Could you check a few things on this drawing? It's one solid part, dimensions in mm from its lowest x, y, z. A direction names the side the tool comes from. Give positions to 0.01 mm unless a question says otherwise; leave off trailing zeros. Order: outer loops, then holes, each group sorted by start corner. A loop starts at its lowest first (then second) coordinate and runs counter-clockwise, first axis right, second up. Notation, with made-up numbers: (14.5, -39.5) - (35.5, -39.5) arc R6 ccw to (35.5, -35.5) - close; hole circle Ø4 at (-29, -38.75). An arc over 180 degrees is marked (long way). One line per question, with ' | ' between items. Start each with the question number.
1. I need wall thicknesses on probe 1 along X at (y, z) = (2.85, 5.1); probe 2 along Z at (x, y) = (5.1, 0.2). Which ranges of each line are inside material? Lowest first, please. Write a range as from..to.
2. Imagine slicing it at B-B (z = 5.1). Please give me the cut outline in (x, y).
3. Imagine slicing it at A-A (x = 5.1). Please give me the cut outline in (y, z), and give its area (3 significant figures).
4. If we mould it in two halves opening along Z, with no side actions, what happens to the marked faces 1, 2 and 3? For each: released by +Z, released by -Z, zero draft, split by the parting line, or undercut.
5. Which directions (+Z, -Z, +X, -X, +Y, -Y) give clear straight access to the entire face, cutting with the end or side of a thin tool? Please do the marked faces 4 and 5.
6. Imagine slicing it at D-D (z = 8.5). Please give me the cut outline in (x, y), and give its area (3 significant figures).
7. Imagine slicing it at C-C (y = 0.6). Please give me the cut outline in (x, z).
8. For P1, Ø3, axis at x = 4.5, z = 5.5, coming from the -Y side; P2, Ø1.5, axis at x = 2, y = 1.5, coming from the -Z side; P3, Ø1, axis at x = 3, z = 7.5, coming from the -Y side; P4, Ø1, axis at y = 2.5, z = 7.5, coming from the +X side, each with a flat end and sliding along its axis, tell me the tip position at first contact or that it passes through.
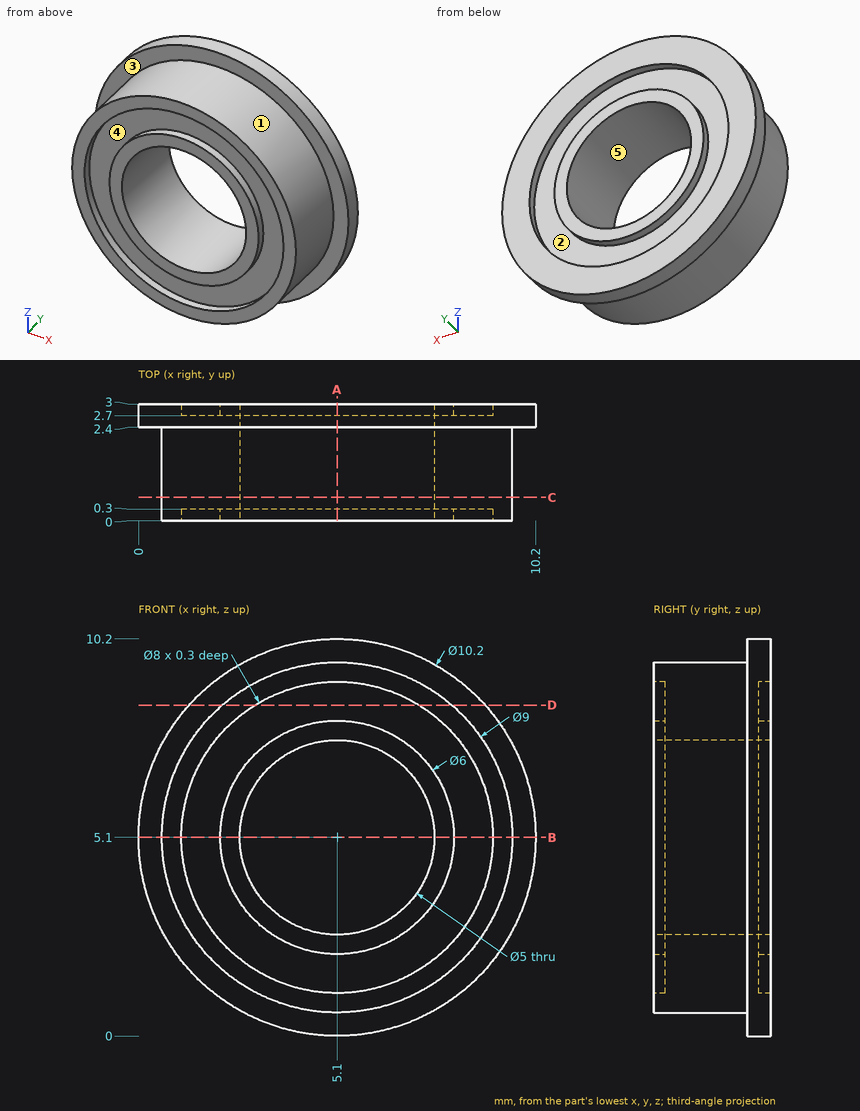
Results found:
1) probe 1: x = 0..1.1, 2.1..2.6, 7.6..8.1, 9.1..10.2 | probe 2: z = 0.6..1.1, 2.1..2.6, 7.6..8.1, 9.1..9.6
2) outline: (0, 2.4) - (0.6, 2.4) - (0.6, 0) - (1.1, 0) - (1.1, 0.3) - (2.1, 0.3) - (2.1, 0) - (2.6, 0) - (2.6, 3) - (2.1, 3) - (2.1, 2.7) - (1.1, 2.7) - (1.1, 3) - (0, 3) - close; (7.6, 0) - (8.1, 0) - (8.1, 0.3) - (9.1, 0.3) - (9.1, 0) - (9.6, 0) - (9.6, 2.4) - (10.2, 2.4) - (10.2, 3) - (9.1, 3) - (9.1, 2.7) - (8.1, 2.7) - (8.1, 3) - (7.6, 3) - close
3) outline: (0, 0.6) - (2.4, 0.6) - (2.4, 0) - (3, 0) - (3, 1.1) - (2.7, 1.1) - (2.7, 2.1) - (3, 2.1) - (3, 2.6) - (0, 2.6) - (0, 2.1) - (0.3, 2.1) - (0.3, 1.1) - (0, 1.1) - close; (0, 7.6) - (3, 7.6) - (3, 8.1) - (2.7, 8.1) - (2.7, 9.1) - (3, 9.1) - (3, 10.2) - (2.4, 10.2) - (2.4, 9.6) - (0, 9.6) - (0, 9.1) - (0.3, 9.1) - (0.3, 8.1) - (0, 8.1) - close | area: 11.5 mm2
4) face 1: split by the parting line | face 2: undercut | face 3: zero draft
5) face 4: -Y | face 5: +Y, -Y
6) outline: (1.3, 2.4) - (2.15, 2.4) - (2.15, 0) - (2.99, 0) - (2.99, 0.3) - (7.21, 0.3) - (7.21, 0) - (8.05, 0) - (8.05, 2.4) - (8.9, 2.4) - (8.9, 3) - (7.21, 3) - (7.21, 2.7) - (2.99, 2.7) - (2.99, 3) - (1.3, 3) - close | area: 16.2 mm2
7) outline: circle Ø9 at (5.1, 5.1); hole circle Ø5 at (5.1, 5.1)
8) P1: passes through | P2: stops at z = 1.26 | P3: stops at y = 0 | P4: stops at x = 9.83
